The listing builds one solid part. Answer for the finished solid, in the listing's coordinates (mm). Face numbers are marked on the shaded views. A direction names the side the tool comes from. Coordinates: 2 decimals unless noted, no trailing zeros. Order: outer loops, then holes, each group sorted by start corner. A loop starts at its lowest first (then second) coordinate and runs counter-clockwise, first axis right, second up. Notation, with made-up numbers: M -31,39.5 L -22,39.5 A12 ccw -22,49.5 Z; hole C 59.25,-24 d5. An arc over 180 degrees is marked long. One line per item, written item: value. Start each with the question number.
Q1. The part is cut by section A-A on y = 0. Give the vertices of the cut face in (x, z), then the cut area to 3 significant figures.
Q2. The part is cut by section B-B on z = 4.75. Give the vertices of the cut face in (x, y).
Q3. Straight lines are drawn through the part: line 1 along Z through (x, y) = (-1, 2.5); line 2 along Z through (x, y) = (0, 0.5); line 3 along Y through (x, z) = (-1, 26.75). For each, find the intervals that lie inside material, in ascending order. Write a range as [from, to].
Q4. Determine the mould class of the marked faces 3, 4 and 5 for opening direction Y: pulls with the +Y half, pulls with the -Y half, needs draft (parallel to the pull), parting line crosses it, or undercut.
Q5. Each of these flat-tipped pins is pushed along its axis until it touches: pin 1 Ø3 at (x, z) = (0, 19.5) entering from -Y; pin 2 Ø1.5 at (y, z) = (0, 9) entering from +X; pin 3 Ø3 at (x, z) = (3, 10) entering from -Y. Where does it stop, or does it pass through?
Q6. For the marked faces 1 and 2, determine the directions among +Z, -Z, +X, -X, +Y, -Y from which every point of the face is accessible in a straight line to the end or side of a thin tool.
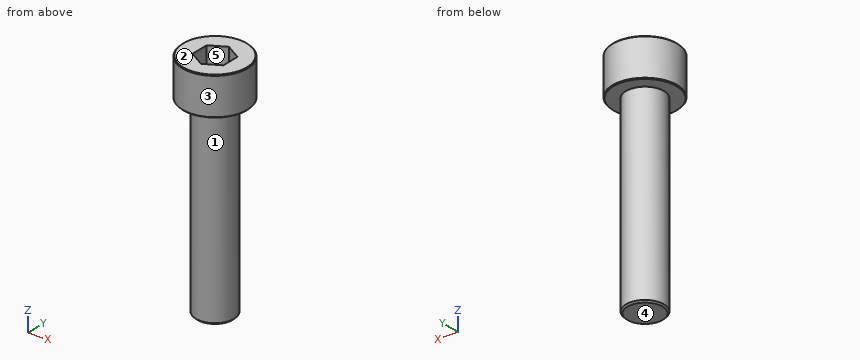
```python
from build123d import *

# Parameters (mm, degrees)
SKETCH_1_W          = 4.25
SKETCH_1_H          = 5
SKETCH_2_R          = 2.5
EXTRUDE_1_DEPTH     = 25
CUT_EXTRUDE_1_DEPTH = 3.75
CHAMFER_1_SIZE2     = 0.100002106
CHAMFER_1_SIZE      = 0.100002056
CHAMFER_2_SIZE      = 0.200033753
CHAMFER_2_SIZE2     = 0.200036689


with BuildPart() as part:
    # 草图1 → 旋转1 (revolve)
    with BuildSketch(Plane(origin=(0, 0, 0), x_dir=(1, 0, 0), z_dir=(0, 1, 0))):
        with Locations((2.125, -27.5)):
            Rectangle(SKETCH_1_W, SKETCH_1_H)
    revolve(axis=Axis((0, 0, 25), (0, 0, 1)))

    # 草图2 → 凸台-拉伸1 (add)
    with BuildSketch(Plane(origin=(0, 0, 25), x_dir=(-1, 0, 0), z_dir=(0, 0, -1))):
        Circle(SKETCH_2_R)
    extrude(amount=EXTRUDE_1_DEPTH)

    # 草图3 → 切除-拉伸1 (cut)
    with BuildSketch(Plane.XY.offset(30)):
        Polygon((-2.01, -1.160474041), (0, -2.320948082), (2.01, -1.160474041), (2.01, 1.160474041), (0, 2.320948082), (-2.01, 1.160474041), align=None)
    extrude(amount=-CUT_EXTRUDE_1_DEPTH, mode=Mode.SUBTRACT)

    # 倒角1
    chamfer_1_edges = [part.edges().sort_by_distance(p)[0] for p in [
        (-4.25, 0, 30),
        (-4.25, 0, 25),
    ]]
    chamfer(chamfer_1_edges, length=CHAMFER_1_SIZE, length2=CHAMFER_1_SIZE2)

    # 倒角2
    chamfer_2_edges = [part.edges().sort_by_distance(p)[0] for p in [
        (2.5, 0, 0),
    ]]
    chamfer_2_side = [part.faces().sort_by_distance(p)[0] for p in [
        (2.5, 0, 12.5),
    ]]
    chamfer(chamfer_2_edges, length=CHAMFER_2_SIZE, length2=CHAMFER_2_SIZE2, reference=chamfer_2_side[0])


solid = part.part
```
Output:
1. outline: M -4.25,25.1 L -4.15,25 L -2.5,25 L -2.5,0.2 L -2.3,0 L 2.3,0 L 2.5,0.2 L 2.5,25 L 4.15,25 L 4.25,25.1 L 4.25,29.9 L 4.15,30 L 2.01,30 L 2.01,26.25 L -2.01,26.25 L -2.01,30 L -4.15,30 L -4.25,29.9 Z
1. area: 152 mm^2
2. outline: C 0,0 d5
3. line 1: z = [25, 30]
3. line 2: z = [0, 26.25]
3. line 3: y = [-4.13, -1.74], [1.74, 4.13]
4. face 3: parting line crosses it
4. face 4: needs draft
4. face 5: undercut
5. pin 1: stops at y = -2.5
5. pin 2: stops at x = 2.5
5. pin 3: stops at y = -2
6. face 1: -Z
6. face 2: +Z, +X, -X, +Y, -Y
